The model under review builds one solid part; all positions refer to its coordinate system, in mm. A direction names the side the tool comes from. Round coordinates to 2 decimals unless told otherwise and drop trailing zeros. Loops run counter-clockwise (first coordinate to the right, second up) from the corner with the lowest first, then second, coordinate; pieces in that order, holes last. Notation, with made-up numbers: (66, 8.5) - (91, 8.5) arc R20 cw to (91, 33.5) - close; hole circle Ø7 at (36, 12). An arc over 180 degrees is marked (long way). Answer as CSV lines item,"result".
from build123d import *

# Parameters (mm, degrees)
SKETCH1_R           = 1.5
BOSS_EXTRUDE1_DEPTH = 11
SKETCH2_R           = 1.5
BOSS_EXTRUDE2_DEPTH = 6
BOSS_EXTRUDE3_DEPTH = 2


with BuildPart() as part:
    # Sketch1 → Boss-Extrude1 (new body)
    with BuildSketch(Plane(origin=(0, 0, 0), x_dir=(0, 0, -1), z_dir=(1, 0, 0))):
        Polygon((1.327905619, 2.3), (-1.327905619, 2.3), (-2.655811238, 0), (-1.327905619, -2.3), (1.327905619, -2.3), (2.655811238, 0), align=None)
        Circle(SKETCH1_R, mode=Mode.SUBTRACT)
    extrude(amount=BOSS_EXTRUDE1_DEPTH)



with BuildPart() as body_2:
    # Sketch2 → Boss-Extrude2 (new body)
    with BuildSketch(Plane(origin=(11, 0, 0), x_dir=(0, 0, -1), z_dir=(1, 0, 0))):
        Circle(SKETCH2_R)
    extrude(amount=BOSS_EXTRUDE2_DEPTH)


with BuildPart() as part_1:
    add(part.part)

    add(body_2.part)  # Boss-Extrude3 merges body 2
    # Sketch3 → Boss-Extrude3 (add)
    with BuildSketch(Plane.ZY.offset(-11)):
        Polygon((-1.327905619, 2.3), (-2.655811238, 0), (-1.327905619, -2.3), (1.327905619, -2.3), (2.655811238, 0), (1.327905619, 2.3), align=None)
    extrude(amount=BOSS_EXTRUDE3_DEPTH)


solid = part_1.part
1. Tool access review of faces 5 (the face through (17, 0, 0)), 6 (the face through (11, 2, 0)): name each direction out of +Z, -Z, +X, -X, +Y, -Y from which nothing blocks a thin tool from reaching the whole face with its end or side.
Numbers:
face 5,"+Z, -Z, +X, +Y, -Y"
face 6,"+X"
2. Take a section at C-C (y = -0.5). State the section outline as (x, z) points.
Numbers:
outline,"(0, -2.37) - (11, -2.37) - (11, -1.41) - (17, -1.41) - (17, 1.41) - (11, 1.41) - (11, 2.37) - (0, 2.37) - (0, 1.41) - (9, 1.41) - (9, -1.41) - (0, -1.41) - close"
3. Take a section at A-A (x = 7). State the section outline as (y, z) points, plus the area to 3 significant figures.
Numbers:
outline,"(-2.3, -1.33) - (0, -2.66) - (2.3, -1.33) - (2.3, 1.33) - (0, 2.66) - (-2.3, 1.33) - close; hole circle Ø3 at (0, 0)"
area,"11.3 mm²"
4. Take a section at B-B (z = 0). State the section outline as (x, y) points.
Numbers:
outline,"(0, -2.3) - (11, -2.3) - (11, -1.5) - (17, -1.5) - (17, 1.5) - (11, 1.5) - (11, 2.3) - (0, 2.3) - (0, 1.5) - (9, 1.5) - (9, -1.5) - (0, -1.5) - close"
5. Take a section at D-D (x = 14.5). State the section outline as (y, z) points, plus the area to 3 significant figures.
Numbers:
outline,"circle Ø3 at (0, 0)"
area,"7.07 mm²"
6. Draft analysis for pull direction Y (two halves, no side actions). For faces 1 (the face through (0, 2, 0)), 2 (the face through (4.44, 0.07, 1.5)), 3 (the face through (13.96, 0.07, 1.5)), 4 (the face through (9, 0, 0)), state which applies: +Y half, -Y half, draft (parallel to the pull), parting line (faces both ways), or undercut.
Numbers:
face 1,"draft"
face 2,"undercut"
face 3,"parting line"
face 4,"undercut"
7. Wall thickness on probe 1 along Y at (x, z) = (2.75, 0); probe 2 along X at (y, z) = (1.9, -0.3); probe 3 along X at (y, z) = (-1, 0.4): over which ranges is each line inside the solid? List them lowest first.
Numbers:
probe 1,"y = -2.3 to -1.5, 1.5 to 2.3"
probe 2,"x = 0 to 11"
probe 3,"x = 9 to 17"
